```python
from build123d import *

# Parameters (mm, degrees)
BOSS_EXTRU_1_DEPTH           = 4
ESQUISSE2_R                  = 1.65
ENL_V_MAT_EXTRU_1_DEPTH      = 2
ESQUISSE3_W                  = 5
ESQUISSE3_H                  = 13
ENL_V_MAT_EXTRU_2_DEPTH      = 20.899748742
ESQUISSE4_W                  = 2.75
ESQUISSE4_H                  = 5.994249795
ESQUISSE4_H_2                = 6.005750205
BOSS_EXTRU_2_DEPTH           = 2
CHANFREIN3_SIZE              = 1.8
CHANFREIN3_OF_SYM_TRIE1_SIZE = 1.8


with BuildPart() as part:
    # Esquisse1 → Boss.-Extru.1 (new body)
    with BuildSketch(Plane.XY):
        with BuildLine():
            Line((12, -14), (-12, -14))
            ThreePointArc((-12, -14), (-13.414213562, -13.414213562), (-14, -12))
            Line((-14, -12), (-14, 12))
            ThreePointArc((-14, 12), (-13.414213562, 13.414213562), (-12, 14))
            Line((-12, 14), (12, 14))
            ThreePointArc((12, 14), (13.414213562, 13.414213562), (14, 12))
            Line((14, 12), (14, -12))
            ThreePointArc((14, -12), (13.414213562, -13.414213562), (12, -14))
        make_face()
    extrude(amount=BOSS_EXTRU_1_DEPTH)

    # Esquisse2 → Enlèv. mat.-Extru.1 (cut)
    with BuildSketch(Plane.XY.offset(4)):
        with BuildLine():
            Line((-10, -12), (10, -12))
            ThreePointArc((10, -12), (11.414213562, -11.414213562), (12, -10))
            Line((12, -10), (12, -9))
            Line((12, -9), (14, -9))
            Line((14, -9), (14, -7))
            Line((14, -7), (13, -7))
            Line((13, -7), (13, -1.005750205))
            Line((13, -1.005750205), (14, -1.005750205))
            Line((14, -1.005750205), (14, 0.994249795))
            Line((14, 0.994249795), (13, 0.994249795))
            Line((13, 0.994249795), (13, 6.988499589))
            Line((13, 6.988499589), (14, 6.988499589))
            Line((14, 6.988499589), (14, 8.988499589))
            Line((14, 8.988499589), (12, 8.988499589))
            Line((12, 8.988499589), (12, 10))
            ThreePointArc((12, 10), (11.414213562, 11.414213562), (10, 12))
            Line((10, 12), (-10, 12))
            ThreePointArc((-10, 12), (-11.414213562, 11.414213562), (-12, 10))
            Line((-12, 10), (-12, 8.988499589))
            Line((-12, 8.988499589), (-14, 8.988499589))
            Line((-14, 8.988499589), (-14, 6.988499589))
            Line((-14, 6.988499589), (-13, 6.988499589))
            Line((-13, 6.988499589), (-13, 0.994249795))
            Line((-13, 0.994249795), (-14, 0.994249795))
            Line((-14, 0.994249795), (-14, -1.005750205))
            Line((-14, -1.005750205), (-13, -1.005750205))
            Line((-13, -1.005750205), (-13, -7))
            Line((-13, -7), (-14, -7))
            Line((-14, -7), (-14, -9))
            Line((-14, -9), (-12, -9))
            Line((-12, -9), (-12, -10))
            ThreePointArc((-12, -10), (-11.414213562, -11.414213562), (-10, -12))
        make_face()
        with Locations((-8.25, 8.25)):
            Circle(ESQUISSE2_R, mode=Mode.SUBTRACT)
        with Locations((8.255750205, 8.244249795)):
            Circle(ESQUISSE2_R, mode=Mode.SUBTRACT)
        with Locations((8.25, -8.261500411)):
            Circle(ESQUISSE2_R, mode=Mode.SUBTRACT)
        with Locations((-8.255750205, -8.255750205)):
            Circle(ESQUISSE2_R, mode=Mode.SUBTRACT)
    extrude(amount=-ENL_V_MAT_EXTRU_1_DEPTH, mode=Mode.SUBTRACT)

    # Esquisse3 → Enlèv. mat.-Extru.2 (cut, through all)
    with BuildSketch(Plane.XY.offset(2)):
        with Locations((-7.5, 0)):
            Rectangle(ESQUISSE3_W, ESQUISSE3_H)
        with Locations((7.5, 0)):
            Rectangle(ESQUISSE3_W, ESQUISSE3_H)
    extrude(amount=-ENL_V_MAT_EXTRU_2_DEPTH, mode=Mode.SUBTRACT)

    # Esquisse4 → Boss.-Extru.2 (add)
    with BuildSketch(Plane.XY.offset(4)):
        with Locations((-12.625, -4.002875103)):
            Rectangle(ESQUISSE4_W, ESQUISSE4_H)
        with Locations((-12.625, 3.997124897)):
            Rectangle(ESQUISSE4_W, ESQUISSE4_H_2)
    boss_extru_2 = extrude(amount=BOSS_EXTRU_2_DEPTH)

    # Chanfrein3
    chanfrein3_edges = [part.edges().sort_by_distance(p)[0] for p in [
        (-11.25, 3.997124897, 6),
        (-11.25, -4.002875103, 6),
    ]]
    chamfer(chanfrein3_edges, length=CHANFREIN3_SIZE)

    # Symétrie1: Boss.-Extru.2 across plane
    add(boss_extru_2.mirror(Plane(origin=(0, 0, 0), x_dir=(0, 0, 1), z_dir=(1, 0, 0))))

    # Chanfrein3 of Symétrie1
    chanfrein3_of_sym_trie1_edges = [part.edges().sort_by_distance(p)[0] for p in [
        (11.25, 3.997124897, 6),
        (11.25, -4.002875103, 6),
    ]]
    chamfer(chanfrein3_of_sym_trie1_edges, length=CHANFREIN3_OF_SYM_TRIE1_SIZE)


solid = part.part
```
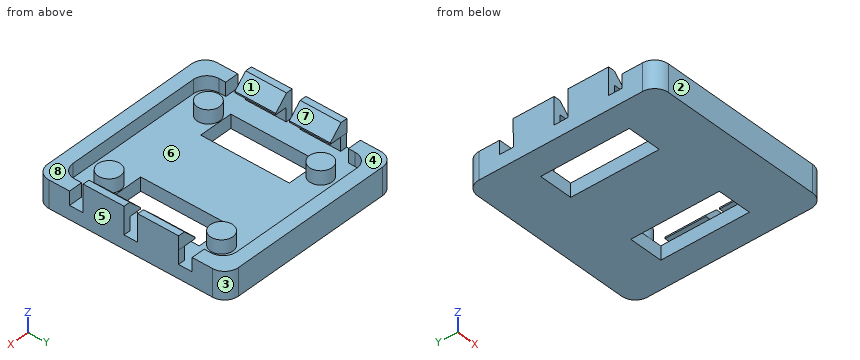
Input: part model. Units: mm. Frame: model coordinates. Face numbers are marked on the shaded views. A direction names the side the tool comes from. Coordinates: 2 decimals unless noted, no trailing zeros. Loops run counter-clockwise (first coordinate to the right, second up) from the corner with the lowest first, then second, coordinate; pieces in that order, holes last. Notation, with made-up numbers: (86.5, 27.5) - (138.5, 27.5) arc R10 ccw to (138.5, 31.5) - close; hole circle Ø5 at (37, -15). An arc over 180 degrees is marked (long way). Answer in a Markdown table with one row per item.
(1) Mould query, pull axis X, two halves, no side actions, for the marked faces 1, 2 and 3. Classes: pulls with the +X half, pulls with the -X half, needs draft (parallel to the pull), parting line crosses it, or undercut.
Model answer:
| item | result |
|---|---|
| face 1 | undercut |
| face 2 | needs draft |
| face 3 | pulls with the +X half |
(2) Cut plane C-C on y = -1.75. Output: boundary loops of the cut face in (x, z), plus the area to 3 significant figures.
Model answer:
| item | result |
|---|---|
| outline | (-14, 0) - (-10, 0) - (-10, 2) - (-13, 2) - (-13, 4) - (-11.25, 4) - (-11.25, 4.2) - (-13.05, 6) - (-14, 6) - close; (-5, 0) - (5, 0) - (5, 2) - (-5, 2) - close; (10, 0) - (14, 0) - (14, 6) - (13.05, 6) - (11.25, 4.2) - (11.25, 4) - (13, 4) - (13, 2) - (10, 2) - close |
| area | 47.8 mm² |
(3) Cut plane A-A on z = 1.4. Output: boundary loops of the cut face in (x, y).
Model answer:
| item | result |
|---|---|
| outline | (-14, -12) arc R2 ccw to (-12, -14) - (12, -14) arc R2 ccw to (14, -12) - (14, 12) arc R2 ccw to (12, 14) - (-12, 14) arc R2 ccw to (-14, 12) - close; hole (-10, -6.5) - (-5, -6.5) - (-5, 6.5) - (-10, 6.5) - close; hole (5, -6.5) - (10, -6.5) - (10, 6.5) - (5, 6.5) - close |
(4) Cut plane D-D on x = -3.5. Output: boundary loops of the cut face in (y, z).
Model answer:
| item | result |
|---|---|
| outline | (-14, 0) - (14, 0) - (14, 4) - (12, 4) - (12, 2) - (-12, 2) - (-12, 4) - (-14, 4) - close |
(5) Cut plane B-B on x = 5.5. Output: boundary loops of the cut face in (y, z).
Model answer:
| item | result |
|---|---|
| outline | (-14, 0) - (-6.5, 0) - (-6.5, 2) - (-12, 2) - (-12, 4) - (-14, 4) - close; (6.5, 0) - (14, 0) - (14, 4) - (12, 4) - (12, 2) - (6.5, 2) - close |
(6) Material intervals for L1, parallel to X at y = -6, z = 1.25; L2, parallel to Y at x = -5, z = 3.15; L3, parallel to Y at x = -5.5, z = 1.3, sorted ascending. Write a range as from..to.
Model answer:
| item | result |
|---|---|
| L1 | x = -14..-10, -5..5, 10..14 |
| L2 | y = -14..-12, 12..14 |
| L3 | y = -14..-6.5, 6.5..14 |
(7) Set-up query: the marked faces 4, 5, 6, 7 and 8. Return all of +Z, -Z, +X, -X, +Y, -Y with unobstructed straight access to the full face (end or side cutting, diameter ignored); none if empty.
Model answer:
| item | result |
|---|---|
| face 4 | +Z, +X, -X, +Y |
| face 5 | +Z, -Z, +X, +Y, -Y |
| face 6 | none |
| face 7 | +Z, +Y, -Y |
| face 8 | +Z, +X, -X, -Y |
(8) Pin query (flat end, axial travel): P1, Ø0.5, axis at x = -13.5, z = 2.5, coming from the +Y side; P2, Ø3.5, axis at x = 8, y = -7.5, coming from the +Z side; P3, Ø1, axis at x = -13, z = 3, coming from the +Y side. Return the tip coordinate at first contact, or that it passes through.
Model answer:
| item | result |
|---|---|
| P1 | stops at y = 13.56 |
| P2 | stops at z = 4 |
| P3 | stops at y = 13.94 |
